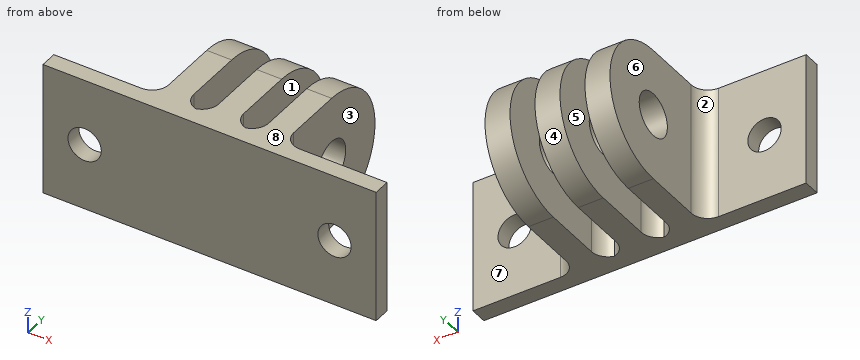
```python
from build123d import *

# Parameters (mm, degrees)
SKETCH_1_W                 = 40
SKETCH_1_H                 = 16
SKETCH_1_R                 = 2
EXTRUDE_1_DEPTH            = 2
SKETCH_2_R                 = 2.6
EXTRUDE_2_DEPTH            = 1.5
PATTERN_LINEAR_1_COUNT     = 2
PATTERN_LINEAR_1_PITCH     = 6
PATTERN_LINEAR_1_COL_COUNT = 2
PATTERN_LINEAR_1_COL_PITCH = 6
FILLET_1_R                 = 2


with BuildPart() as part:
    # 草圖1 → 填料-伸長1 (new body)
    with BuildSketch(Plane(origin=(0, 0, 0), x_dir=(1, 0, 0), z_dir=(0, 1, 0))):
        Rectangle(SKETCH_1_W, SKETCH_1_H)
        with Locations(Location((-15, 0, 0), (0, 0, 270))):
            Circle(SKETCH_1_R, mode=Mode.SUBTRACT)
        with Locations(Location((15, 0, 0), (0, 0, 90))):
            Circle(SKETCH_1_R, mode=Mode.SUBTRACT)
    extrude(amount=EXTRUDE_1_DEPTH)

    # 草圖2 → 填料-伸長2 (add, symmetric)
    with BuildSketch(Plane(origin=(0, 0, 0), x_dir=(0, 0, -1), z_dir=(1, 0, 0))):
        with BuildLine():
            Line((8, 2), (-8, 2))
            Line((-8, 2), (-8, 11))
            ThreePointArc((-8, 11), (0, 19), (8, 11))
            Line((8, 11), (8, 2))
        make_face()
        with Locations((0, 11)):
            Circle(SKETCH_2_R, mode=Mode.SUBTRACT)
    extrude_2 = extrude(amount=EXTRUDE_2_DEPTH, both=True)

    # 直線複製排列1: 填料-伸長2 ×2
    with Locations(*[(i * PATTERN_LINEAR_1_PITCH, 0, 0) for i in range(1, PATTERN_LINEAR_1_COUNT)]):
        add(extrude_2)

    # 直線複製排列1 col: 填料-伸長2 ×2
    with Locations(*[(-i * PATTERN_LINEAR_1_COL_PITCH, 0, 0) for i in range(1, PATTERN_LINEAR_1_COL_COUNT)]):
        add(extrude_2)

    # 圓角1
    # the kernel refuses this fillet: 2 mm, written as the material it adds along each edge
    with BuildSketch(Plane(origin=(1.5, 2, -8), x_dir=(0, 1, 0), z_dir=(0, 0, 1)), Plane(origin=(-1.5, 2, -8), x_dir=(-1, 0, 0), z_dir=(0, 0, 1)), Plane(origin=(-7.5, 2, -8), x_dir=(-1, 0, 0), z_dir=(0, 0, 1)), Plane(origin=(7.5, 2, -8), x_dir=(0, 1, 0), z_dir=(0, 0, 1)), Plane(origin=(4.5, 2, -8), x_dir=(-1, 0, 0), z_dir=(0, 0, 1))) as fillet_1_piece_1:
        with BuildLine():
            CenterArc((FILLET_1_R, -FILLET_1_R), FILLET_1_R, 90, 90)
            Line((0, -FILLET_1_R), (0, 0))
            Line((0, 0), (FILLET_1_R, 0))
        make_face()
    extrude(amount=16)
    with BuildSketch(Plane(origin=(-4.5, 2, -8), x_dir=(1, 0, 0), z_dir=(0, 0, 1))) as fillet_1_piece_2:
        with BuildLine():
            CenterArc((FILLET_1_R, FILLET_1_R), FILLET_1_R, 180, 90)
            Line((0, FILLET_1_R), (0, 0))
            Line((0, 0), (FILLET_1_R, 0))
        make_face()
    extrude(amount=16)


solid = part.part
```
Verification items for the finished model (mm, model axes). Face numbers are marked on the shaded views. A direction names the side the tool comes from. Give positions to 0.01 mm unless a question says otherwise; leave off trailing zeros. Order: outer loops, then holes, each group sorted by start corner. A loop starts at its lowest first (then second) coordinate and runs counter-clockwise, first axis right, second up. Notation, with made-up numbers: M 12.25,25.25 L 49.25,25.25 A16 ccw 49.25,31.25 Z; hole C 57.5,5 d9. An arc over 180 degrees is marked long. Return JSON: item names as keys, results as strings. Group by question number.
1) Section check C-C on y = 12. Record the cut outline in (x, z), and give its area (3 significant figures).
2) Section check D-D on z = 0. Give the number of separate pieces and of enclosed holes in the cut face, and give its area (3 significant figures).
3) Section check B-B on y = 6.5. Record the cut outline in (x, z).
4) Go/stop test with flat-tipped pins: pin 1 Ø4.5 at (y, z) = (15, 1.5) entering from -X; pin 2 Ø2 at (x, y) = (-11, 3.5) entering from +Z; pin 3 Ø1.5 at (x, y) = (-6, 15) entering from +Z; pin 4 Ø8.5 at (x, z) = (16, 4) entering from +Y. Record where each tip stops, or that it passes through.
5) Mould release check, pull along X, two halves, no side actions. Record for the marked faces 1, 2 and 3: pulls with the +X half, pulls with the -X half, needs draft (parallel to the pull), parting line crosses it, or undercut.
6) Access from +Z, -Z, +X, -X, +Y, -Y to the whole of each face (thin tool, end or side, straight path). Record for the marked faces 4, 5, 6, 7 and 8.
7) Section check A-A on x = -15. Record the cut outline in (y, z), and give its area (3 significant figures).
8) Scan lines: line 1 (X direction, y = 1.55, z = 0); line 2 (X direction, y = 4.75, z = -2.25); line 3 (Y direction, x = 12, z = -1). Record each from-to range of solid material in increasing order.
Answer block:
{
 "1": {"outline": "M -7.5,-7.94 L -4.5,-7.94 L -4.5,-2.4 L -7.5,-2.4 Z; M -7.5,2.4 L -4.5,2.4 L -4.5,7.94 L -7.5,7.94 Z; M -1.5,-7.94 L 1.5,-7.94 L 1.5,-2.4 L -1.5,-2.4 Z; M -1.5,2.4 L 1.5,2.4 L 1.5,7.94 L -1.5,7.94 Z; M 4.5,-7.94 L 7.5,-7.94 L 7.5,-2.4 L 4.5,-2.4 Z; M 4.5,2.4 L 7.5,2.4 L 7.5,7.94 L 4.5,7.94 Z", "area": "99.7 mm^2"},
 "2": {"separate pieces": "6", "enclosed holes": "0", "area": "175 mm^2"},
 "3": {"outline": "M -7.5,-8 L -4.5,-8 L -4.5,8 L -7.5,8 Z; M -1.5,-8 L 1.5,-8 L 1.5,8 L -1.5,8 Z; M 4.5,-8 L 7.5,-8 L 7.5,8 L 4.5,8 Z"},
 "4": {"pin 1": "stops at x = -7.5", "pin 2": "passes through", "pin 3": "stops at z = 7.31", "pin 4": "stops at y = 2"},
 "5": {"face 1": "undercut", "face 2": "pulls with the -X half", "face 3": "pulls with the +X half"},
 "6": {"face 4": "+X, -X, +Y", "face 5": "+Z, -Z, +Y", "face 6": "+Z, -Z, -X, +Y", "face 7": "+Z, -Z, +X, +Y", "face 8": "+Z, +X, -X, +Y, -Y"},
 "7": {"outline": "M 0,-8 L 2,-8 L 2,-2 L 0,-2 Z; M 0,2 L 2,2 L 2,8 L 0,8 Z", "area": "24.0 mm^2"},
 "8": {"line 1": "x = -20 to -17, -13 to 13, 17 to 20", "line 2": "x = -7.5 to -4.5, -1.5 to 1.5, 4.5 to 7.5", "line 3": "y = 0 to 2"}
}
